Build history of the part. All positions in model axes, mm. A direction names the side the tool comes from. Give positions to 0.01 mm unless a question says otherwise; leave off trailing zeros. Loops run counter-clockwise (first coordinate to the right, second up) from the corner with the lowest first, then second, coordinate; pieces in that order, holes last. Notation, with made-up numbers: (74.5, 28.25) -> (108.5, 28.25) arc R11 cw to (108.5, 45.25) -> close; hole circle Ø8 at (-27, 15). An arc over 180 degrees is marked (long way). Answer in a Markdown table with one row per item. Add a question column.
from build123d import *

# Parameters (mm, degrees)
SKETCH1_R                    = 1.2
BOSS_EXTRUDE1_DEPTH          = 35
SKETCH2_W                    = 26
SKETCH2_H                    = 10
CUT_EXTRUDE1_DEPTH           = 303.359058075
BOSS_EXTRUDE2_DEPTH          = 7.5
SKETCH4_W                    = 20
SKETCH4_H                    = 26
CUT_EXTRUDE2_DEPTH           = 303.359058075
BOSS_EXTRUDE3_START          = 17.5
SKETCH6_R                    = 3.6
BOSS_EXTRUDE3_DEPTH          = 15
M3_CLEARANCE_HOLE1_OUTLINE_R = 1.8
M3_CLEARANCE_HOLE1_DEPTH     = 4
CUT_EXTRUDE7_DEPTH           = 303.359058075
FILLET8_R                    = 4


# Read off the part's stored shape, not the designer's step: M3 Clearance Hole1
with BuildPart() as part:
    # Sketch1 → Boss-Extrude1 (new, symmetric)
    with BuildSketch(Plane.XY):
        with BuildLine():
            Line((0, 0), (300, 0))
            Line((300, 0), (300, 4))
            ThreePointArc((300, 4), (295.545227279, 5.845227279), (293.7, 10.3))
            ThreePointArc((293.7, 10.3), (290, 14), (286.3, 10.3))
            ThreePointArc((286.3, 10.3), (284.454772721, 5.845227279), (280, 4))
            Line((280, 4), (20, 4))
            ThreePointArc((20, 4), (15.545227279, 5.845227279), (13.7, 10.3))
            ThreePointArc((13.7, 10.3), (10, 14), (6.3, 10.3))
            ThreePointArc((6.3, 10.3), (4.454772721, 5.845227279), (0, 4))
            Line((0, 4), (0, 0))
        make_face()
        with Locations((10, 10.3)):
            Circle(SKETCH1_R, mode=Mode.SUBTRACT)
        with Locations((290, 10.3)):
            Circle(SKETCH1_R, mode=Mode.SUBTRACT)
    extrude(amount=BOSS_EXTRUDE1_DEPTH, both=True)

    # Sketch2 → Cut-Extrude1 (cut, through all)
    with BuildSketch(Plane(origin=(0, 0, 0), x_dir=(0, 0, -1), z_dir=(1, 0, 0))):
        with Locations((0, 9)):
            Rectangle(SKETCH2_W, SKETCH2_H)
    extrude(amount=CUT_EXTRUDE1_DEPTH, mode=Mode.SUBTRACT)

    # Sketch3 → Boss-Extrude2 (add, symmetric)
    with BuildSketch(Plane.XY):
        with BuildLine():
            Line((284, 18), (264, 18))
            ThreePointArc((264, 18), (254.100505063, 13.899494937), (250, 4))
            Line((250, 4), (284, 4))
            ThreePointArc((284, 4), (280, 8), (284, 12))
            ThreePointArc((284, 12), (287, 15), (284, 18))
        make_face()
    extrude(amount=BOSS_EXTRUDE2_DEPTH, both=True)

    # Sketch4 → Cut-Extrude2 (cut, through all)
    with BuildSketch(Plane(origin=(0, 4, 0), x_dir=(1, 0, 0), z_dir=(0, 1, 0))):
        with Locations((10, 0)):
            Rectangle(SKETCH4_W, SKETCH4_H)
    extrude(amount=-CUT_EXTRUDE2_DEPTH, mode=Mode.SUBTRACT)

    # Sketch6 → Boss-Extrude3 (add)
    with BuildSketch(Plane(origin=(0, 0, 0), x_dir=(0, 0, -1), z_dir=(1, 0, 0)).offset(BOSS_EXTRUDE3_START)):
        with BuildLine():
            Line((-14.487917861, 4), (-5.57596765, 9.781748355))
            ThreePointArc((-5.57596765, 9.781748355), (0, 4.7), (5.57596765, 9.781748355))
            Line((5.57596765, 9.781748355), (14.487917861, 4))
            Line((14.487917861, 4), (20, 4))
            Line((20, 4), (3.047850082, 14.997936768))
            ThreePointArc((3.047850082, 14.997936768), (0, 15.9), (-3.047850082, 14.997936768))
            Line((-3.047850082, 14.997936768), (-20, 4))
            Line((-20, 4), (-14.487917861, 4))
        make_face()
        with Locations((0, 10.3)):
            Circle(SKETCH6_R, mode=Mode.SUBTRACT)
    extrude(amount=BOSS_EXTRUDE3_DEPTH)

    # M3 Clearance Hole1 outline → M3 Clearance Hole1 (cut)
    with BuildSketch(Plane(origin=(0, 0, 0), x_dir=(1, 0, 0), z_dir=(0, 1, 0))):
        with Locations((30, -30)):
            Circle(M3_CLEARANCE_HOLE1_OUTLINE_R)
        with Locations((270, 30)):
            Circle(M3_CLEARANCE_HOLE1_OUTLINE_R)
        with Locations((270, -30)):
            Circle(M3_CLEARANCE_HOLE1_OUTLINE_R)
        with Locations((30, 30)):
            Circle(M3_CLEARANCE_HOLE1_OUTLINE_R)
    extrude(amount=M3_CLEARANCE_HOLE1_DEPTH, mode=Mode.SUBTRACT)

    # Sketch12 → Cut-Extrude7 (cut, through all)
    with BuildSketch(Plane(origin=(0, 4, 0), x_dir=(1, 0, 0), z_dir=(0, 1, 0))):
        Polygon((53.630917429, -29), (138.25, -29), (138.25, -3.136996028), align=None)
        Polygon((38.5, -27.350626478), (127.986315, 0), (38.5, 27.350626478), align=None)
        Polygon((138.25, 3.136996028), (138.25, 29), (53.630917429, 29), align=None)
        Polygon((144.25, 29), (144.25, 3.136996028), (228.869082571, 29), align=None)
        Polygon((154.513685, 0), (244, -27.350626478), (244, 27.350626478), align=None)
        Polygon((144.25, -29), (228.869082571, -29), (144.25, -3.136996028), align=None)
    extrude(amount=-CUT_EXTRUDE7_DEPTH, mode=Mode.SUBTRACT)

    # Fillet8
    fillet8_edges = [part.edges().sort_by_distance(p)[0] for p in [
        (53.630917429, 2, -29),
        (138.25, 2, -29),
        (138.25, 2, -3.136996028),
        (38.5, 2, 27.350626478),
        (38.5, 2, -27.350626478),
        (127.986315, 2, 0),
        (244, 2, 27.350626478),
        (154.513685, 2, 0),
        (244, 2, -27.350626478),
        (144.25, 2, -29),
        (228.869082571, 2, -29),
        (144.25, 2, -3.136996028),
        (144.25, 2, 29),
        (144.25, 2, 3.136996028),
        (228.869082571, 2, 29),
        (53.630917429, 2, 29),
        (138.25, 2, 3.136996028),
        (138.25, 2, 29),
    ]]
    fillet(fillet8_edges, radius=FILLET8_R)


solid = part.part
(1) Two-plate mould, pull along Y, no slides. Class faces 1 (the flat face through (24.89, 6.93, -9.97)), 2 (the flat face through (10, 6, -13)), 3 (the cylindrical face through (4.5, 5.89, -23.85)): released by +Y, released by -Y, zero draft, split by the parting line, or undercut.
(2) Wall check: line 1 along X through (y, z) = (10.3, 30.75); line 2 along X through (y, z) = (2.5, -2); line 3 along X through (y, z) = (11.25, 29). Give the ranges that are in metal, low to high. Write a range as from..to.
(3) Saw through at B-B, the plane x = 65.5. List the corners of the cut face in (y, z), then the cut area to 3 significant figures.
(4) Saw through at C-C, the plane x = 199. List the corners of the cut face in (y, z).
(5) Saw through at A-A, the plane z = 0. List the corners of the cut face in (x, y).
(6) 3-axis set-ups, long thin cutter, end or side, ignore diameter. For faces 4 (the flat face through (148, 0, 0)), 5 (the flat face through (203.43, 2.03, -14.95)), 6 (the flat face through (24.895, 6.85, 10.094)), 7 (the flat face through (290, 8, -13)), 8 (the flat face through (32.5, 6, 2)): which of +Z, -Z, +X, -X, +Y, -Y reach the whole face in a straight line?
(7) Flat gauge pins, fed straight in: pin 1 Ø4 at (x, y) = (91.5, 7.5) entering from -Z; pin 2 Ø5.5 at (y, z) = (8, -5.5) entering from -X; pin 3 Ø8 at (y, z) = (15, -14.5) entering from +X; pin 4 Ø1.2 at (y, z) = (2.5, 4.5) entering from -X. Where does each tip first touch, or does it go through?
Worked answers:
| question | item | result |
|---|---|---|
| 1 | face 1 | undercut |
| 1 | face 2 | zero draft |
| 1 | face 3 | released by +Y |
| 2 | line 1 | 6.3..8.8, 11.2..13.7, 286.3..288.8, 291.2..293.7 |
| 2 | line 2 | 20..38.5, 117.77..164.73, 244..300 |
| 2 | line 3 | 6.42..9.27, 10.73..13.58, 286.42..289.27, 290.73..293.58 |
| 3 | outline | (0, -35) -> (4, -35) -> (4, -19.1) -> (0, -19.1) -> close; (0, 19.1) -> (4, 19.1) -> (4, 35) -> (0, 35) -> close |
| 3 | area | 127 mm^2 |
| 4 | outline | (0, -35) -> (4, -35) -> (4, -29) -> (0, -29) -> close; (0, -19.87) -> (4, -19.87) -> (4, -13.6) -> (0, -13.6) -> close; (0, 13.6) -> (4, 13.6) -> (4, 19.87) -> (0, 19.87) -> close; (0, 29) -> (4, 29) -> (4, 35) -> (0, 35) -> close |
| 5 | outline | (17.5, 4.7) -> (32.5, 4.7) -> (32.5, 6.7) -> (17.5, 6.7) -> close; (17.5, 13.9) -> (32.5, 13.9) -> (32.5, 15.9) -> (17.5, 15.9) -> close; (20, 0) -> (38.5, 0) -> (38.5, 4) -> (20, 4) -> close; (118.3, 0) -> (164.2, 0) -> (164.2, 4) -> (118.3, 4) -> close; (244, 0) -> (300, 0) -> (300, 4) -> (284, 4) arc R4 cw to (284, 12) arc R3 ccw to (284, 18) -> (264, 18) arc R14 ccw to (250, 4) -> (244, 4) -> close |
| 6 | face 4 | +Z, -Z, +X, -X, -Y |
| 6 | face 5 | +Y, -Y |
| 6 | face 6 | none |
| 6 | face 7 | +X, +Y |
| 6 | face 8 | +Z, -Z, +Y |
| 7 | pin 1 | through |
| 7 | pin 2 | x = 17.5 |
| 7 | pin 3 | x = 293.63 |
| 7 | pin 4 | x = 20 |
